Can you work these out from the model? Positions are in its coordinate system, mm. Round coordinates to 2 decimals unless told otherwise and drop trailing zeros. Order: outer loops, then holes, each group sorted by start corner. A loop starts at its lowest first (then second) coordinate and runs counter-clockwise, first axis right, second up. Notation, with made-up numbers: (30.5, -24) -> (67.5, -24) arc R15 cw to (67.5, 5) -> close; hole circle Ø1 at (-36.75, 12). An arc over 180 degrees is marked (long way). One line per item, written item: value.
```python
from build123d import *

# Parameters (mm, degrees)
SKETCH1_W           = 133.35
SKETCH1_H           = 117.475
SKETCH1_R           = 14.2748
SKETCH1_R_2         = 9.525
SKETCH1_R_3         = 2.0193
SKETCH1_R_4         = 14.2875
SKETCH1_R_5         = 4.064
SKETCH1_R_6         = 2.667
BOSS_EXTRUDE1_DEPTH = 3.175
FILLET1_R           = 6.35


with BuildPart() as part:
    # Sketch1 → Boss-Extrude1 (new, symmetric)
    with BuildSketch(Plane.XY):
        with Locations((0, 21.6789)):
            Rectangle(SKETCH1_W, SKETCH1_H)
        with Locations((0, 40.7162)):
            Circle(SKETCH1_R, mode=Mode.SUBTRACT)
        with Locations((33.0581, 40.7162)):
            Circle(SKETCH1_R_2, mode=Mode.SUBTRACT)
        with Locations((-33.0581, 40.7162)):
            Circle(SKETCH1_R_2, mode=Mode.SUBTRACT)
        with Locations((-33.0581, 66.1162)):
            Circle(SKETCH1_R_3, mode=Mode.SUBTRACT)
        with Locations((-33.0581, 15.3162)):
            Circle(SKETCH1_R_3, mode=Mode.SUBTRACT)
        Circle(SKETCH1_R_4, mode=Mode.SUBTRACT)
        with Locations((-57.15, 70.8914)):
            Circle(SKETCH1_R_5, mode=Mode.SUBTRACT)
        with Locations((-55.626, -30.2006)):
            Circle(SKETCH1_R_5, mode=Mode.SUBTRACT)
        with Locations((57.15, 70.8914)):
            Circle(SKETCH1_R_5, mode=Mode.SUBTRACT)
        with Locations((55.626, -30.2006)):
            Circle(SKETCH1_R_5, mode=Mode.SUBTRACT)
        with Locations((38.6588, -18.3134)):
            Circle(SKETCH1_R_6, mode=Mode.SUBTRACT)
        with Locations((-38.6588, -18.3134)):
            Circle(SKETCH1_R_6, mode=Mode.SUBTRACT)
        with Locations((33.0581, 66.1162)):
            Circle(SKETCH1_R_3, mode=Mode.SUBTRACT)
        with Locations((33.0581, 15.3162)):
            Circle(SKETCH1_R_3, mode=Mode.SUBTRACT)
    extrude(amount=BOSS_EXTRUDE1_DEPTH, both=True)

    # Fillet1
    fillet1_edges = [part.edges().sort_by_distance(p)[0] for p in [
        (66.675, -37.0586, 0),
        (-66.675, -37.0586, 0),
        (-66.675, 80.4164, 0),
        (66.675, 80.4164, 0),
    ]]
    fillet(fillet1_edges, radius=FILLET1_R)


solid = part.part
```
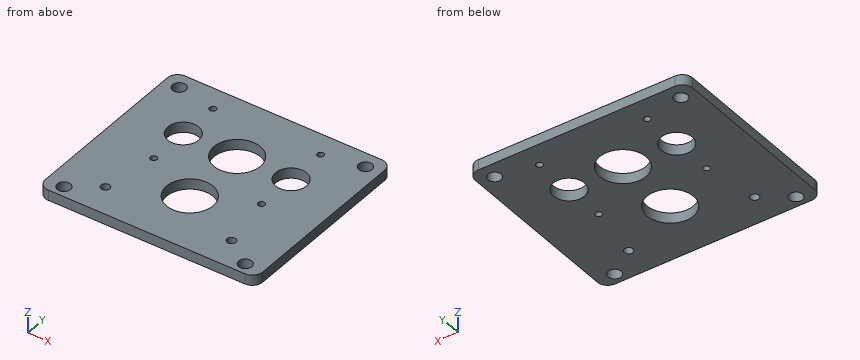
Q1. I want a section at B-B on y = 0. List the corners of the cut face in (x, z) for me (1 decimal), plus the area to 3 significant figures.
Answers below:
outline: (-66.7, -3.2) -> (-14.3, -3.2) -> (-14.3, 3.2) -> (-66.7, 3.2) -> close; (14.3, -3.2) -> (66.7, -3.2) -> (66.7, 3.2) -> (14.3, 3.2) -> close
area: 665 mm^2
Q2. I want a section at A-A on x = 0. List the corners of the cut face in (y, z) for me (1 decimal).
Answers below:
outline: (-37.1, -3.2) -> (-14.3, -3.2) -> (-14.3, 3.2) -> (-37.1, 3.2) -> close; (14.3, -3.2) -> (26.4, -3.2) -> (26.4, 3.2) -> (14.3, 3.2) -> close; (55, -3.2) -> (80.4, -3.2) -> (80.4, 3.2) -> (55, 3.2) -> close
Q3. I want a section at D-D on y = -28.5. List the corners of the cut face in (x, z) for me (3 decimals).
Answers below:
outline: (-66.675, -3.175) -> (-59.317, -3.175) -> (-59.317, 3.175) -> (-66.675, 3.175) -> close; (-51.935, -3.175) -> (51.935, -3.175) -> (51.935, 3.175) -> (-51.935, 3.175) -> close; (59.317, -3.175) -> (66.675, -3.175) -> (66.675, 3.175) -> (59.317, 3.175) -> close
Q4. I want a section at C-C on z = 0.25. Give the number of separate pieces and of enclosed holes in the cut face, plus the area to 3 significant figures.
Answers below:
separate pieces: 1
enclosed holes: 14
area: 13,500 mm^2
Q5. Please list where these lines run through material, in increasing order: line 1 along Y through (x, z) = (0, 0.75); line 2 along X through (y, z) = (41, 0) (3 decimals); line 3 along Y through (x, z) = (-40, 0.5).
Answers below:
line 1: -37.06 to -14.29, 14.29 to 26.44, 54.99 to 80.42
line 2: -66.675 to -42.579, -23.537 to -14.272, 14.272 to 23.537, 42.579 to 66.675
line 3: -37.06 to -20.62, -16.01 to 34.19, 47.24 to 80.42
Q6. Will these pins go through, and if not, where does the flat tip stop? pin 1 Ø17 at (x, y) = (-33.06, 40.72) entering from +Z; pin 2 Ø13 at (x, y) = (57.15, 70.89) entering from -Z (3 decimals).
Answers below:
pin 1: through
pin 2: z = -3.175
